Build history of the part. All positions in model axes, mm. A direction names the side the tool comes from. Give positions to 0.01 mm unless a question says otherwise; leave off trailing zeros. Order: outer loops, then holes, each group sorted by start corner. A loop starts at its lowest first (then second) coordinate and runs counter-clockwise, first axis right, second up. Notation, with made-up numbers: (36.5, -5.75) - (49.5, -5.75) arc R29 cw to (49.5, 31.25) - close; hole circle Ø6 at (77.5, 58.25). An arc over 180 degrees is marked (long way). Write each question's results on one line, items separated by ' | '. Start each with the question number.
1) Cut at C-C on y = 4. List the corners of the cut face in (x, z), plus the area to 3 significant figures.
2) Cut at B-B on x = -6.25. List the corners of the cut face in (y, z), plus the area to 3 significant figures.
3) Two-plate mould, pull along Y, no slides. Class faces 1 (the face through (3.755, 5.423, -11.923)), 2 (the face through (7, 0, -11)), 3 (the face through (10, 9, 10)): +Y half, -Y half, draft (parallel to the pull), parting line (faces both ways), or undercut.
4) Cut at A-A on z = 0. List the corners of the cut face in (x, y), plus the area to 3 significant figures.
5) Drill centre lines: line 1 along X through (y, z) = (6.25, 0); line 2 along Y through (x, z) = (13.25, -4.5); line 3 along Z through (x, y) = (10.75, 3.75). Where is each one in solid material? Low to high. Write a range as from..to.
6) Tool access for faces 4 (the face through (10, 2, -10)), 5 (the face through (-5.554, 0.986, 13.394)): list every direction of +Z, -Z, +X, -X, +Y, -Y with a clear straight run to the whole face (end or side of a thin tool).
7) Drop flat-ended pins along their axis: pin 1 Ø6 at (x, z) = (-11, 11) entering from +Y; pin 2 Ø6 at (x, z) = (8.5, 0.5) entering from +Y; pin 3 Ø1 at (y, z) = (5.5, -10.5) entering from +X. Give the stop position or say it passes through.
from build123d import *

# Parameters (mm, degrees)
SKETCH1_R           = 14.5
BOSS_EXTRUDE1_DEPTH = 11
SKETCH2_R           = 12.5
CUT_EXTRUDE1_DEPTH  = 24.270152556


with BuildPart() as part:
    # Sketch1 → Boss-Extrude1 (new body)
    with BuildSketch(Plane(origin=(0, 0, 0), x_dir=(1, 0, 0), z_dir=(0, 1, 0))):
        with Locations(Location((0, 0, 0), (0, 0, 270))):
            Circle(SKETCH1_R)
    extrude(amount=BOSS_EXTRUDE1_DEPTH)

    # Sketch2 → Cut-Extrude1 (cut, through all)
    with BuildSketch(Plane.XZ):
        with Locations(Location((0, 0, 0), (0, 0, 270))):
            Circle(SKETCH2_R)
    extrude(amount=-CUT_EXTRUDE1_DEPTH, mode=Mode.SUBTRACT)

    # Sketch3 → Cut-Revolve2 (revolve, cut)
    with BuildSketch(Plane(origin=(0, 0, 0), x_dir=(0, 0, -1), z_dir=(1, 0, 0))):
        Polygon((-14.5, 11), (-14.5, 9), (-13.5, 9), (-13.5, 2), (-14.5, 2), (-14.5, 0), (-16.729305882, 5.995742764), align=None)
    revolve(axis=Axis((0, 11.640939065, 0), (0, -1, 0)), mode=Mode.SUBTRACT)


solid = part.part
Results:
1) outline: circle Ø27 at (0, 0); hole circle Ø25 at (0, 0) | area: 81.7 mm^2
2) outline: (0, -13.08) - (2, -13.08) - (2, -11.97) - (9, -11.97) - (9, -13.08) - (11, -13.08) - (11, -10.83) - (0, -10.83) - close; (0, 10.83) - (11, 10.83) - (11, 13.08) - (9, 13.08) - (9, 11.97) - (2, 11.97) - (2, 13.08) - (0, 13.08) - close | area: 34.0 mm^2
3) face 1: draft | face 2: -Y half | face 3: undercut
4) outline: (-14.5, 0) - (-12.5, 0) - (-12.5, 11) - (-14.5, 11) - (-14.5, 9) - (-13.5, 9) - (-13.5, 2) - (-14.5, 2) - close; (12.5, 0) - (14.5, 0) - (14.5, 2) - (13.5, 2) - (13.5, 9) - (14.5, 9) - (14.5, 11) - (12.5, 11) - close | area: 30.0 mm^2
5) line 1: -13.5..-12.5, 12.5..13.5 | line 2: 0..2, 9..11 | line 3: -8.17..-6.38, 6.38..8.17
6) face 4: none | face 5: +Y, -Y
7) pin 1: y = 11 | pin 2: through | pin 3: x = 9.07
